Geometry check sheet. Reference: the model listing, model coordinates, mm. Face numbers are marked on the shaded views. Give positions to 0.01 mm unless a question says otherwise; leave off trailing zeros. Order: outer loops, then holes, each group sorted by start corner. A loop starts at its lowest first (then second) coordinate and runs counter-clockwise, first axis right, second up. Notation, with made-up numbers: M 15,70.25 L 32,70.25 A34 ccw 32,104.25 Z; hole C 53,34 d8. An arc over 180 degrees is marked long. Answer as CSV lines item,"result".
from build123d import *

# Parameters (mm, degrees)
SKETCH1_W               = 107
SKETCH1_H               = 107
BOSS_EXTRUDE1_DEPTH     = 6
SHELL6_T                = -2
CUT_EXTRUDE1_DEPTH      = 151.03332963
CUT_EXTRUDE1_DEPTH_BACK = 105
SKETCH2_W               = 89
SKETCH2_H               = 3
CUT_EXTRUDE2_DEPTH      = 152.439756999
CUT_EXTRUDE2_DEPTH_BACK = 152.439756999
SKETCH3_W               = 4.823716506
SKETCH3_H               = 87
SKETCH4_R               = 1.75
BOSS_EXTRUDE2_DEPTH     = 7
BOSS_EXTRUDE3_START     = 3
SKETCH5_R               = 1.75
BOSS_EXTRUDE3_DEPTH     = 3
SKETCH6_W               = 127
SKETCH6_H               = 127
CUT_EXTRUDE3_DEPTH      = 3
FILLET2_R               = 3


with BuildPart() as part:
    # Sketch1 → Boss-Extrude1 (new body)
    with BuildSketch(Plane.XY):
        with Locations((53.5, 53.5)):
            Rectangle(SKETCH1_W, SKETCH1_H)
    extrude(amount=BOSS_EXTRUDE1_DEPTH)

    # Shell6
    shell6_openings = [part.faces().sort_by_distance(p)[0] for p in [
        (53.5, 53.5, 0),
    ]]
    offset(amount=SHELL6_T, openings=shell6_openings, kind=Kind.INTERSECTION)

    # Sketch2 → Cut-Extrude1 (cut, two sides: drawn at the far end of the back side and taken through both)
    with BuildSketch(Plane.XZ.offset(-105).offset(-CUT_EXTRUDE1_DEPTH_BACK)):
        with Locations((54.5, 1.5)):
            Rectangle(SKETCH2_W, SKETCH2_H)
    extrude(amount=CUT_EXTRUDE1_DEPTH + CUT_EXTRUDE1_DEPTH_BACK, mode=Mode.SUBTRACT)

    # Sketch3 → Cut-Extrude2 (cut, two sides: drawn at the far end of the back side and taken through both)
    with BuildSketch(Plane(origin=(107, 0, 0), x_dir=(0, 0, -1), z_dir=(1, 0, 0)).offset(-CUT_EXTRUDE2_DEPTH_BACK)):
        with Locations((-0.588141747, 53.5)):
            Rectangle(SKETCH3_W, SKETCH3_H)
    extrude(amount=CUT_EXTRUDE2_DEPTH + CUT_EXTRUDE2_DEPTH_BACK, mode=Mode.SUBTRACT)

    # Sketch4 → Boss-Extrude2 (add)
    # profile 1 of 4: a face of its own
    with BuildSketch(Plane.XY.offset(6)):
        Polygon((10, 107), (10, 97), (-10, 97), (-10, 117), (10, 117), align=None)
        with Locations((-1.5, 108.5)):
            Circle(SKETCH4_R, mode=Mode.SUBTRACT)
    # profile 2 of 4: a face of its own
    with BuildSketch(Plane.XY.offset(6)):
        Polygon((97, 97), (117, 97), (117, 117), (97, 117), (97, 107), align=None)
        with Locations(Location((108.5, 108.5, 0), (0, 0, 180))):
            Circle(SKETCH4_R, mode=Mode.SUBTRACT)
    # profile 3 of 4: a face of its own
    with BuildSketch(Plane.XY.offset(6)):
        Polygon((117, -10), (97, -10), (97, 0), (97, 10), (117, 10), align=None)
        with Locations((108.5, -1.5)):
            Circle(SKETCH4_R, mode=Mode.SUBTRACT)
    # profile 4 of 4: a face of its own
    with BuildSketch(Plane.XY.offset(6)):
        Polygon((10, 0), (10, 10), (-10, 10), (-10, -10), (10, -10), align=None)
        with Locations(Location((-1.5, -1.5, 0), (0, 0, 180))):
            Circle(SKETCH4_R, mode=Mode.SUBTRACT)
    extrude(amount=BOSS_EXTRUDE2_DEPTH)

    # Sketch5 → Boss-Extrude3 (add)
    # profile 1 of 4: a face of its own
    with BuildSketch(Plane(origin=(0, 0, 6), x_dir=(-1, 0, 0), z_dir=(0, 0, -1)).offset(BOSS_EXTRUDE3_START)):
        Polygon((-107, 97), (-117, 97), (-117, 117), (-97, 117), (-97, 107), (-107, 107), align=None)
        with Locations((-108.5, 108.5)):
            Circle(SKETCH5_R, mode=Mode.SUBTRACT)
    # profile 2 of 4: a face of its own
    with BuildSketch(Plane(origin=(0, 0, 6), x_dir=(-1, 0, 0), z_dir=(0, 0, -1)).offset(BOSS_EXTRUDE3_START)):
        Polygon((10, 97), (10, 117), (-10, 117), (-10, 107), (0, 107), (0, 97), align=None)
        with Locations(Location((1.5, 108.5, 0), (0, 0, 180))):
            Circle(SKETCH5_R, mode=Mode.SUBTRACT)
    # profile 3 of 4: a face of its own
    with BuildSketch(Plane(origin=(0, 0, 6), x_dir=(-1, 0, 0), z_dir=(0, 0, -1)).offset(BOSS_EXTRUDE3_START)):
        Polygon((10, 10), (10, -10), (-10, -10), (-10, 0), (0, 0), (0, 10), align=None)
        with Locations((1.5, -1.5)):
            Circle(SKETCH5_R, mode=Mode.SUBTRACT)
    # profile 4 of 4: a face of its own
    with BuildSketch(Plane(origin=(0, 0, 6), x_dir=(-1, 0, 0), z_dir=(0, 0, -1)).offset(BOSS_EXTRUDE3_START)):
        Polygon((-117, 10), (-117, -10), (-97, -10), (-97, 0), (-107, 0), (-107, 10), align=None)
        with Locations(Location((-108.5, -1.5, 0), (0, 0, 180))):
            Circle(SKETCH5_R, mode=Mode.SUBTRACT)
    extrude(amount=-BOSS_EXTRUDE3_DEPTH)

    # Sketch6 → Cut-Extrude3 (cut)
    with BuildSketch(Plane.XY.offset(13)):
        with Locations((53.5, 53.5)):
            Rectangle(SKETCH6_W, SKETCH6_H)
    extrude(amount=-CUT_EXTRUDE3_DEPTH, mode=Mode.SUBTRACT)

    # Fillet2
    # the kernel refuses this fillet: 3 mm, written as the material it adds along each edge
    with BuildSketch(Plane(origin=(107, 97, 3), x_dir=(0, -1, 0), z_dir=(0, 0, 1)), Plane(origin=(0, 97, 3), x_dir=(-1, 0, 0), z_dir=(0, 0, 1)), Plane(origin=(10, 107, 3), x_dir=(1, 0, 0), z_dir=(0, 0, 1)), Plane(origin=(0, 10, 3), x_dir=(0, 1, 0), z_dir=(0, 0, 1)), Plane(origin=(107, 10, 3), x_dir=(1, 0, 0), z_dir=(0, 0, 1)), Plane(origin=(97, 0, 3), x_dir=(-1, 0, 0), z_dir=(0, 0, 1))) as fillet2_piece_1:
        with BuildLine():
            CenterArc((FILLET2_R, FILLET2_R), FILLET2_R, 180, 90)
            Line((0, FILLET2_R), (0, 0))
            Line((0, 0), (FILLET2_R, 0))
        make_face()
    extrude(amount=3)
    with BuildSketch(Plane(origin=(97, 107, 3), x_dir=(-1, 0, 0), z_dir=(0, 0, 1)), Plane(origin=(10, 0, 3), x_dir=(1, 0, 0), z_dir=(0, 0, 1))) as fillet2_piece_2:
        with BuildLine():
            CenterArc((FILLET2_R, -FILLET2_R), FILLET2_R, 90, 90)
            Line((0, -FILLET2_R), (0, 0))
            Line((0, 0), (FILLET2_R, 0))
        make_face()
    extrude(amount=3)
    # the kernel refuses this fillet: 3 mm, written as the material it takes off along each edge
    with BuildSketch(Plane(origin=(-10, -10, -4.5), x_dir=(1, 0, 0), z_dir=(0, 0, 1)), Plane(origin=(10, -10, -4.5), x_dir=(0, 1, 0), z_dir=(0, 0, 1)), Plane(origin=(-10, 10, 17.5), x_dir=(1, 0, 0), z_dir=(0, 0, -1)), Plane(origin=(97, -10, -4.5), x_dir=(1, 0, 0), z_dir=(0, 0, 1)), Plane(origin=(117, -10, -4.5), x_dir=(0, 1, 0), z_dir=(0, 0, 1)), Plane(origin=(117, 10, -4.5), x_dir=(-1, 0, 0), z_dir=(0, 0, 1)), Plane(origin=(117, 97, -4.5), x_dir=(0, 1, 0), z_dir=(0, 0, 1)), Plane(origin=(10, 117, -4.5), x_dir=(-1, 0, 0), z_dir=(0, 0, 1))) as fillet2_2_piece_1:
        with BuildLine():
            CenterArc((FILLET2_R, FILLET2_R), FILLET2_R, 180, 90)
            Line((0, FILLET2_R), (0, 0))
            Line((0, 0), (FILLET2_R, 0))
        make_face()
    extrude(amount=22, mode=Mode.SUBTRACT)
    with BuildSketch(Plane(origin=(97, 117, 17.5), x_dir=(0, -1, 0), z_dir=(0, 0, -1)), Plane(origin=(117, 117, 17.5), x_dir=(-1, 0, 0), z_dir=(0, 0, -1)), Plane(origin=(-10, 97, 17.5), x_dir=(1, 0, 0), z_dir=(0, 0, -1)), Plane(origin=(-10, 117, 17.5), x_dir=(0, -1, 0), z_dir=(0, 0, -1))) as fillet2_2_piece_2:
        with BuildLine():
            CenterArc((FILLET2_R, -FILLET2_R), FILLET2_R, 90, 90)
            Line((0, -FILLET2_R), (0, 0))
            Line((0, 0), (FILLET2_R, 0))
        make_face()
    extrude(amount=22, mode=Mode.SUBTRACT)


solid = part.part
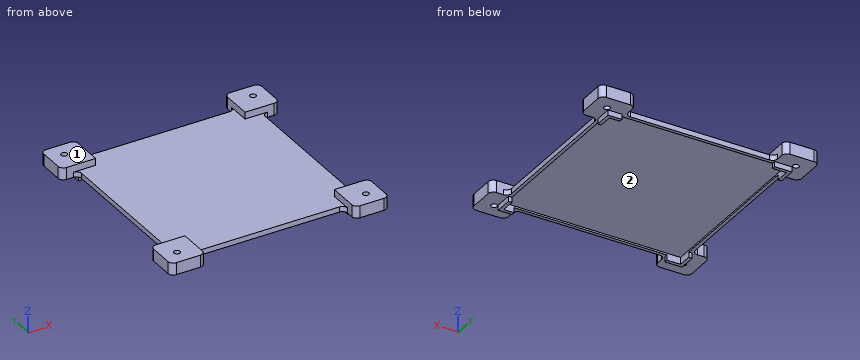
(1) Material ranges on line 1 (Y direction, x = -1.5, z = 7); line 2 (X direction, y = 8, z = 2.75), recorded low to high.
The answers:
line 1,"y = -10 to -3.25, 0.25 to 10, 97 to 106.75, 110.25 to 117"
line 2,"x = 0 to 2, 105 to 107"
(2) Gauge pin test, flat ends, axial feed: P1, Ø1.6, axis at y = 1.5, z = 2, coming from the -X side; P2, Ø2, axis at y = 105.5, z = 1.5, coming from the +X side; P3, Ø6, axis at x = 76.5, z = 2, coming from the -Y side. Record the tip position at first contact, or that the pin passes through.
The answers:
P1,"stops at x = 0"
P2,"stops at x = 107"
P3,"stops at y = 0"
(3) Draft check along X on the marked faces 1 and 2. Enter one of: +X half, -X half, draft (parallel to the pull), parting line (faces both ways), or undercut.
The answers:
face 1,"draft"
face 2,"undercut"
(4) Section check B-B on y = 54. Enter the section's corners in (x, z), then the cut area to 3 significant figures.
The answers:
outline,"M 0,3 L 2,3 L 2,4 L 105,4 L 105,3 L 107,3 L 107,6 L 0,6 Z"
area,"218 mm2"
(5) Section check A-A on y = 108.5. Enter the section's corners in (x, z).
The answers:
outline,"M -10,3 L -3.25,3 L -3.25,10 L -10,10 Z; M 0.25,3 L 10.4,3 L 10.4,6 L 10,6 L 10,10 L 0.25,10 Z; M 96.6,3 L 106.75,3 L 106.75,10 L 97,10 L 97,6 L 96.6,6 Z; M 110.25,3 L 117,3 L 117,10 L 110.25,10 Z"
